Part model, mm, in its own coordinate system. Face numbers are marked on the shaded views. Round coordinates to 2 decimals unless told otherwise and drop trailing zeros. Loops run counter-clockwise (first coordinate to the right, second up) from the corner with the lowest first, then second, coordinate; pieces in that order, holes last. Notation, with made-up numbers: (88.5, -15.75) -> (142.5, -15.75) arc R14 cw to (142.5, 8.25) -> close; hole circle Ø10 at (37.5, 36). An arc over 180 degrees is marked (long way). Use a Markdown table: item, result. Add a question column.
Item 1: Cut at C-C, the plane z = 0. List the corners of the cut face in (x, y), plus the area to 3 significant figures.
Item 2: Flat gauge pins, fed straight in: pin 1 (2 mm diameter, centred on y = -34, z = -1.5, fed in from +X); pin 2 (2 mm diameter, centred on x = 3.5, y = -15.5, fed in from -Z); pin 3 (8.5 mm diameter, centred on x = 21, y = -9.2, fed in from -Z); pin 4 (4 mm diameter, centred on x = 21, y = -34.2, fed in from +Z). Where does each tip first touch, or does it go through?
Item 3: Two-plate mould, pull along Y, no slides. Class the marked faces 1, 2, 3 and 4: pulls with the +Y half, pulls with the -Y half, needs draft (parallel to the pull), parting line crosses it, or undercut.
Item 4: Cut at A-A, the plane y = -9.2. List the corners of the cut face in (x, z), plus the area to 3 significant figures.
Item 5: Cut at B-B, the plane x = 23.5. State how many separate pieces and enclosed holes the cut face has, plus the area to 3 significant figures.
Item 6: Probe line 1 (Y direction, x = 21, z = 2.2); line 2 (Y direction, x = 24, z = 3.25); line 3 (Z direction, x = 25, y = -25). List the from-to ranges inside material, lowest first. Write a range as [from, to].
Item 7: Cut at D-D, the plane y = -25. List the corners of the cut face in (x, z), plus the area to 3 significant figures.
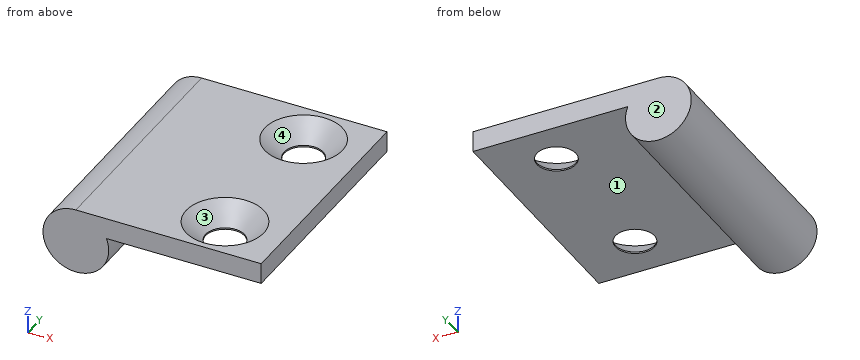
```python
from build123d import *

# Parameters (mm, degrees)
EXTRUDE1_DEPTH       = 40
HOLEWZD1_D           = 6.5
HOLEWZD1_DEPTH       = 11
HOLEWZD1_CSINK_D     = 13
HOLEWZD1_CSINK_ANGLE = 90


with BuildPart() as part:
    # Sketch1 → Extrude1 (new body)
    with BuildSketch(Plane.XZ.offset(41.7)):
        with BuildLine():
            Line((31, 5.5), (0, 5.5))
            ThreePointArc((0, 5.5), (-3.102418411, -4.541475531), (5.123475383, 2))
            Line((5.123475383, 2), (31, 2))
            Line((31, 2), (31, 5.5))
        make_face()
    extrude(amount=-EXTRUDE1_DEPTH)

    # HoleWzd1
    with Locations(Plane.XY.offset(5.5)):
        with Locations((21, -34.2), (21, -9.2)):
            CounterSinkHole(HOLEWZD1_D / 2, HOLEWZD1_CSINK_D / 2, depth=HOLEWZD1_DEPTH, counter_sink_angle=HOLEWZD1_CSINK_ANGLE)


solid = part.part
```
A:
| question | item | result |
|---|---|---|
| 1 | outline | (-5.5, -41.7) -> (5.5, -41.7) -> (5.5, -1.7) -> (-5.5, -1.7) -> close |
| 1 | area | 440 mm^2 |
| 2 | pin 1 | stops at x = 5.48 |
| 2 | pin 2 | stops at z = -4.9 |
| 2 | pin 3 | stops at z = 2 |
| 2 | pin 4 | passes through |
| 3 | face 1 | needs draft |
| 3 | face 2 | pulls with the +Y half |
| 3 | face 3 | undercut |
| 3 | face 4 | undercut |
| 4 | outline | (0, 5.5) arc R5.5 ccw (long way) to (5.12, 2) -> (17.75, 2) -> (17.75, 2.25) -> (14.5, 5.5) -> close; (24.25, 2) -> (31, 2) -> (31, 5.5) -> (27.5, 5.5) -> (24.25, 2.25) -> close |
| 4 | area | 157 mm^2 |
| 5 | separate pieces | 3 |
| 5 | enclosed holes | 0 |
| 5 | area | 84.1 mm^2 |
| 6 | line 1 | y = [-41.7, -37.45], [-30.95, -12.45], [-5.95, -1.7] |
| 6 | line 2 | y = [-41.7, -37.21], [-31.19, -12.21], [-6.19, -1.7] |
| 6 | line 3 | z = [2, 5.5] |
| 7 | outline | (0, 5.5) arc R5.5 ccw (long way) to (5.12, 2) -> (31, 2) -> (31, 5.5) -> close |
| 7 | area | 191 mm^2 |
